Read the model definition and answer for the solid it produces. Units are mm, in the model's axes. A direction names the side the tool comes from. Coordinates: 2 decimals unless noted, no trailing zeros. Loops run counter-clockwise (first coordinate to the right, second up) from the corner with the lowest first, then second, coordinate; pieces in that order, holes last. Notation, with made-up numbers: (-35.75, 72.5) -> (14.25, 72.5) arc R15 ccw to (14.25, 88.5) -> close; hole circle Ø3 at (3, 57). An arc over 180 degrees is marked (long way). Answer as a JSON object with one key per item and string values. Group by question number.
Q1. The part is cut by section B-B on x = 7.5. Write down the section's boundary in (y, z).
Q2. Straight lines are drawn through the part: line 1 along Z through (x, y) = (7.5, 6.25); line 2 along X through (y, z) = (5.5, 2.5); line 3 along Z through (x, y) = (8.75, 5). For each, find the intervals that lie inside material, in ascending order. Write a range as [from, to].
Q3. Each of these flat-tipped pins is pushed along its axis until it touches: P1, Ø12, axis at x = 23.5, y = 17.5, coming from the -Z side; P2, Ø1.5, axis at x = 6.5, y = 18, coming from the -Z side; P3, Ø2, axis at x = 10, y = 10.5, coming from the -Z side. Where does it stop, or does it pass through?
Q4. For faces 1 (the flat face through (22, 15, 4)), 2 (the cylindrical face through (4, 10, 0)), 3 (the flat face through (30, 15, 5)), determine the directions among +Z, -Z, +X, -X, +Y, -Y from which every point of the face is accessible in a straight line to the end or side of a thin tool.
Q5. Determine the mould class of faces 4 (the flat face through (7, 20, 0)), 5 (the flat face through (1, 15, 0)), 6 (the flat face through (15, 15, 2)) for opening direction Z: released by +Z, released by -Z, zero draft, split by the parting line, or undercut.
Q6. The part is cut by section C-C on z = -1.25. Write down the section's boundary in (x, y).
Q7. The part is cut by section A-A on y = 11.75. Write down the section's boundary in (x, z).
Q8. The part is cut by section D-D on x = 18.75. Write down the section's boundary in (y, z), and give its area (3 significant figures).
from build123d import *

# Parameters (mm, degrees)
SKETCH1_W               = 30
SKETCH1_H               = 30
BOSS_EXTRUDE1_DEPTH     = 10
SKETCH2_W               = 15
SKETCH2_H               = 30
CUT_EXTRUDE1_DEPTH      = 4
SKETCH4_R               = 1.75
CUT_EXTRUDE3_DEPTH      = 30
SKETCH7_R               = 5
BOSS_EXTRUDE2_DEPTH     = 40
SKETCH8_R               = 3.5
CUT_EXTRUDE4_DEPTH      = 30
SKETCH9_W               = 3
SKETCH9_H               = 30
CUT_EXTRUDE5_DEPTH      = 31
SKETCH11_W              = 33.170745935
SKETCH11_H              = 13.10963014
CUT_EXTRUDE6_DEPTH      = 6
CUT_EXTRUDE6_DEPTH_BACK = 8
SKETCH12_R              = 3.5
BOSS_EXTRUDE3_DEPTH     = 10
BOSS_EXTRUDE4_DEPTH     = 3


with BuildPart() as part:
    # Sketch1 → Boss-Extrude1 (new body)
    with BuildSketch(Plane.XY):
        with Locations((15, 15)):
            Rectangle(SKETCH1_W, SKETCH1_H)
    extrude(amount=BOSS_EXTRUDE1_DEPTH)

    # Sketch2 → Cut-Extrude1 (cut)
    with BuildSketch(Plane(origin=(0, 0, 0), x_dir=(-1, 0, 0), z_dir=(0, 0, -1))):
        with Locations((-22.5, 15)):
            Rectangle(SKETCH2_W, SKETCH2_H)
    extrude(amount=-CUT_EXTRUDE1_DEPTH, mode=Mode.SUBTRACT)

    # Sketch4 → Cut-Extrude3 (cut)
    with BuildSketch(Plane(origin=(0, 0, 4), x_dir=(-1, 0, 0), z_dir=(0, 0, -1))):
        with Locations((-22.5, 0)):
            Circle(SKETCH4_R)
        with Locations((-22.5, 30)):
            Circle(SKETCH4_R)
    extrude(amount=-CUT_EXTRUDE3_DEPTH, mode=Mode.SUBTRACT)

    # Sketch7 → Boss-Extrude2 (add)
    with BuildSketch(Plane.XZ):
        with Locations((7.5, 0)):
            Circle(SKETCH7_R)
    extrude(amount=-BOSS_EXTRUDE2_DEPTH)

    # Sketch8 → Cut-Extrude4 (cut)
    with BuildSketch(Plane.XZ):
        with Locations((7.5, 0)):
            Circle(SKETCH8_R)
    extrude(amount=-CUT_EXTRUDE4_DEPTH, mode=Mode.SUBTRACT)

    # Sketch9 → Cut-Extrude5 (cut, through all)
    with BuildSketch(Plane.ZY):
        with Locations((8.5, 15)):
            Rectangle(SKETCH9_W, SKETCH9_H)
    extrude(amount=-CUT_EXTRUDE5_DEPTH, mode=Mode.SUBTRACT)

    # Sketch11 → Cut-Extrude6 (cut, two sides)
    with BuildSketch(Plane(origin=(0, 0, 0), x_dir=(-1, 0, 0), z_dir=(0, 0, -1))) as cut_extrude6_sk:
        with Locations((-15.51660734, 36.55481507)):
            Rectangle(SKETCH11_W, SKETCH11_H)
    extrude(amount=CUT_EXTRUDE6_DEPTH, mode=Mode.SUBTRACT)
    extrude(cut_extrude6_sk.sketch, amount=-CUT_EXTRUDE6_DEPTH_BACK, mode=Mode.SUBTRACT)

    # Sketch12 → Boss-Extrude3 (add)
    with BuildSketch(Plane(origin=(0, 30, 0), x_dir=(1, 0, 0), z_dir=(0, 1, 0))):
        with Locations((7.5, 0)):
            Circle(SKETCH12_R)
    extrude(amount=-BOSS_EXTRUDE3_DEPTH)

    # Sketch13 → Boss-Extrude4 (add)
    with BuildSketch(Plane(origin=(0, 0, 4), x_dir=(-1, 0, 0), z_dir=(0, 0, -1))):
        with BuildLine():
            Line((-24.25, 30), (-20.75, 30))
            ThreePointArc((-20.75, 30), (-22.5, 28.25), (-24.25, 30))
        make_face()
        with BuildLine():
            Line((-24.25, 0), (-20.75, 0))
            ThreePointArc((-20.75, 0), (-22.5, 1.75), (-24.25, 0))
        make_face()
    extrude(amount=-BOSS_EXTRUDE4_DEPTH)


solid = part.part
Final values:
{
 "1": {"outline": "(0, -5) -> (30, -5) -> (30, 7) -> (0, 7) -> (0, 3.5) -> (20, 3.5) -> (20, -3.5) -> (0, -3.5) -> close"},
 "2": {"line 1": "z = [-5, -3.5], [3.5, 7]", "line 2": "x = [0, 5.05], [9.95, 15]", "line 3": "z = [-4.84, -3.27], [3.27, 7]"},
 "3": {"P1": "stops at z = 4", "P2": "stops at z = -4.99", "P3": "stops at z = -4.77"},
 "4": {"face 1": "-Z, +X, +Y, -Y", "face 2": "-Y", "face 3": "+Z, -Z, +X, +Y, -Y"},
 "5": {"face 4": "undercut", "face 5": "released by -Z", "face 6": "zero draft"},
 "6": {"outline": "(2.66, 0) -> (4.23, 0) -> (4.23, 20) -> (10.77, 20) -> (10.77, 0) -> (12.34, 0) -> (12.34, 30) -> (2.66, 30) -> close"},
 "7": {"outline": "(0, 0) -> (2.5, 0) arc R5 ccw to (12.5, 0) -> (15, 0) -> (15, 4) -> (30, 4) -> (30, 7) -> (0, 7) -> close; hole circle Ø7 at (7.5, 0)"},
 "8": {"outline": "(0, 4) -> (30, 4) -> (30, 7) -> (0, 7) -> close", "area": "90.0 mm2"}
}
